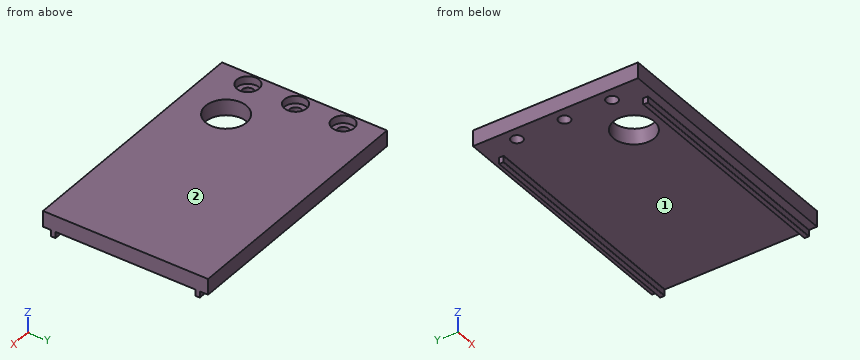
from build123d import *

# Parameters (mm, degrees)
ESQUISSE1_W                                        = 80
ESQUISSE1_H                                        = 52
BOSS_EXTRU_1_DEPTH                                 = 5
ESQUISSE2_R                                        = 6.447859464
ENL_V_MAT_EXTRU_1_DEPTH                            = 5
CHAMBRAGE_POUR_VIS_T_TE_RONDE_BOMB_E_M_D           = 3.6
CHAMBRAGE_POUR_VIS_T_TE_RONDE_BOMB_E_M_CBORE_D     = 7
CHAMBRAGE_POUR_VIS_T_TE_RONDE_BOMB_E_M_CBORE_DEPTH = 2.4
ESQUISSE5_W                                        = 72
ESQUISSE5_H                                        = 1.45
BOSS_EXTRU_2_DEPTH                                 = 2
CONG_1_R                                           = 0.1


with BuildPart() as part:
    # Esquisse1 → Boss.-Extru.1 (new body)
    with BuildSketch(Plane.XY.offset(16.98011664)):
        with Locations((-44.444303066, 24.066569306)):
            Rectangle(ESQUISSE1_W, ESQUISSE1_H)
    extrude(amount=BOSS_EXTRU_1_DEPTH)

    # Esquisse2 → Enlèv. mat.-Extru.1 (cut)
    with BuildSketch(Plane.XY.offset(21.98011664)):
        with Locations((-66.444303066, 12.061734253)):
            Circle(ESQUISSE2_R)
    extrude(amount=-ENL_V_MAT_EXTRU_1_DEPTH, mode=Mode.SUBTRACT)

    # Chambrage pour vis à tête ronde bombée M34 (through all)
    with Locations(Plane.XY.offset(21.98011664)):
        with Locations((-80.444303066, 9.066569306), (-80.444303066, 24.066569306), (-80.444303066, 39.066569306)):
            CounterBoreHole(CHAMBRAGE_POUR_VIS_T_TE_RONDE_BOMB_E_M_D / 2, CHAMBRAGE_POUR_VIS_T_TE_RONDE_BOMB_E_M_CBORE_D / 2, CHAMBRAGE_POUR_VIS_T_TE_RONDE_BOMB_E_M_CBORE_DEPTH)

    # Esquisse5 → Boss.-Extru.2 (add)
    with BuildSketch(Plane(origin=(0, 0, 16.98011664), x_dir=(-1, 0, 0), z_dir=(0, 0, -1))):
        with Locations((40.444303066, 1.341569306)):
            Rectangle(ESQUISSE5_W, ESQUISSE5_H)
        with Locations((40.444303066, 46.791569306)):
            Rectangle(ESQUISSE5_W, ESQUISSE5_H)
    extrude(amount=BOSS_EXTRU_2_DEPTH)

    # Congé1
    cong_1_edges = [part.edges().sort_by_distance(p)[0] for p in [
        (-40.444303066, 0.616569306, 16.98011664),
        (-40.444303066, 2.066569306, 16.98011664),
        (-40.444303066, 0.616569306, 14.98011664),
        (-40.444303066, 2.066569306, 14.98011664),
        (-40.444303066, 46.066569306, 16.98011664),
        (-40.444303066, 47.516569306, 16.98011664),
        (-40.444303066, 46.066569306, 14.98011664),
        (-40.444303066, 47.516569306, 14.98011664),
    ]]
    fillet(cong_1_edges, radius=CONG_1_R)


solid = part.part
Work out the finished part from the listing and answer in its coordinate system (mm). Face numbers are marked on the shaded views. Give positions to 0.01 mm unless a question says otherwise; leave off trailing zeros. Loops run counter-clockwise (first coordinate to the right, second up) from the corner with the lowest first, then second, coordinate; pieces in that order, holes last. Notation, with made-up numbers: (77.5, 38) -> (87.5, 38) arc R21 cw to (87.5, 45) -> close; hole circle Ø10 at (-23, -13). An arc over 180 degrees is marked (long way). Use a Markdown table: item, result. Add a question column.
1) For a pull along Y with two mould halves and no side action, classify the marked faces 1 and 2 as +Y half, -Y half, draft (parallel to the pull), parting line (faces both ways), or undercut.
2) Consider line 1 along Y through (x, z) = (-60.5, 16.5); line 2 along X through (y, z) = (11, 20); line 3 along Z through (x, y) = (-42.5, 30). Determine where each line is inside the solid, lowest interval first.
3) The part is cut by section D-D, the plane z = 20.5. Determine the outline of the cut face in (x, y), plus the area to 3 significant figures.
4) The part is cut by section B-B, the plane y = 6.5. Determine the outline of the cut face in (x, z), plus the area to 3 significant figures.
5) The part is cut by section A-A, the plane x = -68. Determine the outline of the cut face in (y, z).
6) Each of these flat-tipped pins is pushed along its axis until it touches: P1, Ø0.9, axis at x = -55.5, z = 16, coming from the -Y side; P2, Ø6.5, axis at x = -80.44, y = 24.07, coming from the -Z side; P3, Ø1.3, axis at y = 47, z = 16, coming from the -X side; P4, Ø3, axis at x = -80.44, y = 39.07, coming from the -Z side. Where does it stop, or does it pass through?
7) The part is cut by section C-C, the plane x = -58.5. Determine the outline of the cut face in (y, z).
Reported:
| question | item | result |
|---|---|---|
| 1 | face 1 | undercut |
| 1 | face 2 | draft |
| 2 | line 1 | y = 0.62 to 2.07, 46.07 to 47.52 |
| 2 | line 2 | x = -84.44 to -83.36, -77.53 to -72.8, -60.08 to -4.44 |
| 2 | line 3 | z = 16.98 to 21.98 |
| 3 | outline | (-84.44, -1.93) -> (-4.44, -1.93) -> (-4.44, 50.07) -> (-84.44, 50.07) -> close; hole circle Ø7 at (-80.44, 9.07); hole circle Ø7 at (-80.44, 24.07); hole circle Ø7 at (-80.44, 39.07); hole circle Ø12.9 at (-66.44, 12.06) |
| 3 | area | 3,910 mm^2 |
| 4 | outline | (-84.44, 16.98) -> (-69.71, 16.98) -> (-69.71, 21.98) -> (-78.06, 21.98) -> (-78.06, 19.58) -> (-82.82, 19.58) -> (-82.82, 21.98) -> (-84.44, 21.98) -> close; (-63.18, 16.98) -> (-4.44, 16.98) -> (-4.44, 21.98) -> (-63.18, 21.98) -> close |
| 4 | area | 356 mm^2 |
| 5 | outline | (-1.93, 16.98) -> (0.52, 16.98) arc R0.1 cw to (0.62, 16.88) -> (0.62, 15.08) arc R0.1 ccw to (0.72, 14.98) -> (1.97, 14.98) arc R0.1 ccw to (2.07, 15.08) -> (2.07, 16.88) arc R0.1 cw to (2.17, 16.98) -> (5.8, 16.98) -> (5.8, 21.98) -> (-1.93, 21.98) -> close; (18.32, 16.98) -> (45.97, 16.98) arc R0.1 cw to (46.07, 16.88) -> (46.07, 15.08) arc R0.1 ccw to (46.17, 14.98) -> (47.42, 14.98) arc R0.1 ccw to (47.52, 15.08) -> (47.52, 16.88) arc R0.1 cw to (47.62, 16.98) -> (50.07, 16.98) -> (50.07, 21.98) -> (18.32, 21.98) -> close |
| 6 | P1 | stops at y = 0.62 |
| 6 | P2 | stops at z = 16.98 |
| 6 | P3 | stops at x = -76.44 |
| 6 | P4 | passes through |
| 7 | outline | (-1.93, 16.98) -> (0.52, 16.98) arc R0.1 cw to (0.62, 16.88) -> (0.62, 15.08) arc R0.1 ccw to (0.72, 14.98) -> (1.97, 14.98) arc R0.1 ccw to (2.07, 15.08) -> (2.07, 16.88) arc R0.1 cw to (2.17, 16.98) -> (45.97, 16.98) arc R0.1 cw to (46.07, 16.88) -> (46.07, 15.08) arc R0.1 ccw to (46.17, 14.98) -> (47.42, 14.98) arc R0.1 ccw to (47.52, 15.08) -> (47.52, 16.88) arc R0.1 cw to (47.62, 16.98) -> (50.07, 16.98) -> (50.07, 21.98) -> (-1.93, 21.98) -> close |
